The listing builds one solid part. Answer for the finished solid, in the listing's coordinates (mm). Coordinates: 2 decimals unless noted, no trailing zeros. Order: outer loops, then holes, each group sorted by start corner. A loop starts at its lowest first (then second) coordinate and runs counter-clockwise, first axis right, second up. Notation, with made-up numbers: (-14.75, 1) -> (6.25, 1) arc R12 ccw to (6.25, 18) -> close; hole circle Ø7 at (-4.75, -7.75). An arc over 180 degrees is marked (long way). Return JSON: item names as keys, results as strings.
from build123d import *

# Parameters (mm, degrees)
F1_DEPTH = 15
F2_R     = 20
F3_DEPTH = 25
F4_SIZE  = 2


with BuildPart() as f1:
    # F0 (on Front) → F1 (new body)
    with BuildSketch(Plane.XZ):
        Polygon((24.8435035413, 24.90530428), (-0.0436997214, 35.1777193664), (-24.90530428, 24.8435035413), (-35.1777193664, -0.0436997214), (-24.8435035413, -24.90530428), (0.0436997214, -35.1777193664), (24.90530428, -24.8435035413), (35.1777193664, 0.0436997214), align=None)
    extrude(amount=F1_DEPTH)

    # F2 (on face) → F3 (cut)
    with BuildSketch(Plane.XZ.offset(15)):
        Circle(F2_R)
    extrude(amount=-F3_DEPTH, mode=Mode.SUBTRACT)

    # F4
    f4_edges = [f1.edges().sort_by_distance(p)[0] for p in [
        (30.041512, -15, -12.399902),
        (12.474502, -15, -30.010611),
        (30.010611, -15, 12.474502),
        (-12.399902, -15, -30.041512),
        (12.399902, -15, 30.041512),
        (-30.010611, -15, -12.474502),
        (-12.474502, -15, 30.010611),
        (-30.041512, -15, 12.399902),
        (-20, -15, 0),
        (30.041512, 0, -12.399902),
        (12.474502, 0, -30.010611),
        (30.010611, 0, 12.474502),
        (-12.399902, 0, -30.041512),
        (12.399902, 0, 30.041512),
        (-30.010611, 0, -12.474502),
        (-12.474502, 0, 30.010611),
        (-30.041512, 0, 12.399902),
        (-20, 0, 0),
    ]]
    chamfer(f4_edges, length=F4_SIZE)


solid = f1.part
1. Consider line 1 (Z direction, x = 0, y = -5.75); line 2 (X direction, y = -5.75, z = 16); line 3 (X direction, y = -4.5, z = -13.5). Determine where each line is inside the solid, lowest interval first. Write a range as from..to.
Answer block:
{"line 1": "z = -35.16..-20, 20..35.16", "line 2": "x = -28.56..-12, 12..28.55", "line 3": "x = -29.58..-14.76, 14.76..29.59"}
2. Each of these flat-tipped pins is pushed along its axis until it touches: pin 1 Ø1.5 at (y, z) = (-10.5, -19.5) entering from +X; pin 2 Ø2 at (y, z) = (-2.5, -4) entering from +X; pin 3 Ø3 at (x, y) = (-28, -4) entering from -Z. Where does it stop, or does it pass through?
Answer block:
{"pin 1": "stops at x = 27.42", "pin 2": "stops at x = 33.92", "pin 3": "stops at z = -20.92"}
3. Determine the mould class of faces 1 (the face through (11.92, -13.99, -29.17)), 2 (the face through (29.15, -0.99, 11.91)), 3 (the face through (-4.336, -7.577, -19.524)) for opening direction Z: pulls with the +Z half, pulls with the -Z half, needs draft (parallel to the pull), parting line crosses it, or undercut.
Answer block:
{"face 1": "pulls with the -Z half", "face 2": "pulls with the +Z half", "face 3": "undercut"}
4. The part is cut by section B-B on x = 27. Give the vertices of the cut face in (y, z).
Answer block:
{"outline": "(-15, -14.53) -> (-13, -19.77) -> (-2, -19.77) -> (0, -14.53) -> (0, 14.51) -> (-2, 19.72) -> (-13, 19.72) -> (-15, 14.51) -> close"}
5. The part is cut by section A-A on y = -6. Give the vertices of the cut face in (x, z), and give its area (3 significant figures).
Answer block:
{"outline": "(-35.18, -0.04) -> (-24.84, -24.91) -> (0.04, -35.18) -> (24.91, -24.84) -> (35.18, 0.04) -> (24.84, 24.91) -> (-0.04, 35.18) -> (-24.91, 24.84) -> close; hole circle Ø40 at (0, 0)", "area": "2,240 mm2"}
